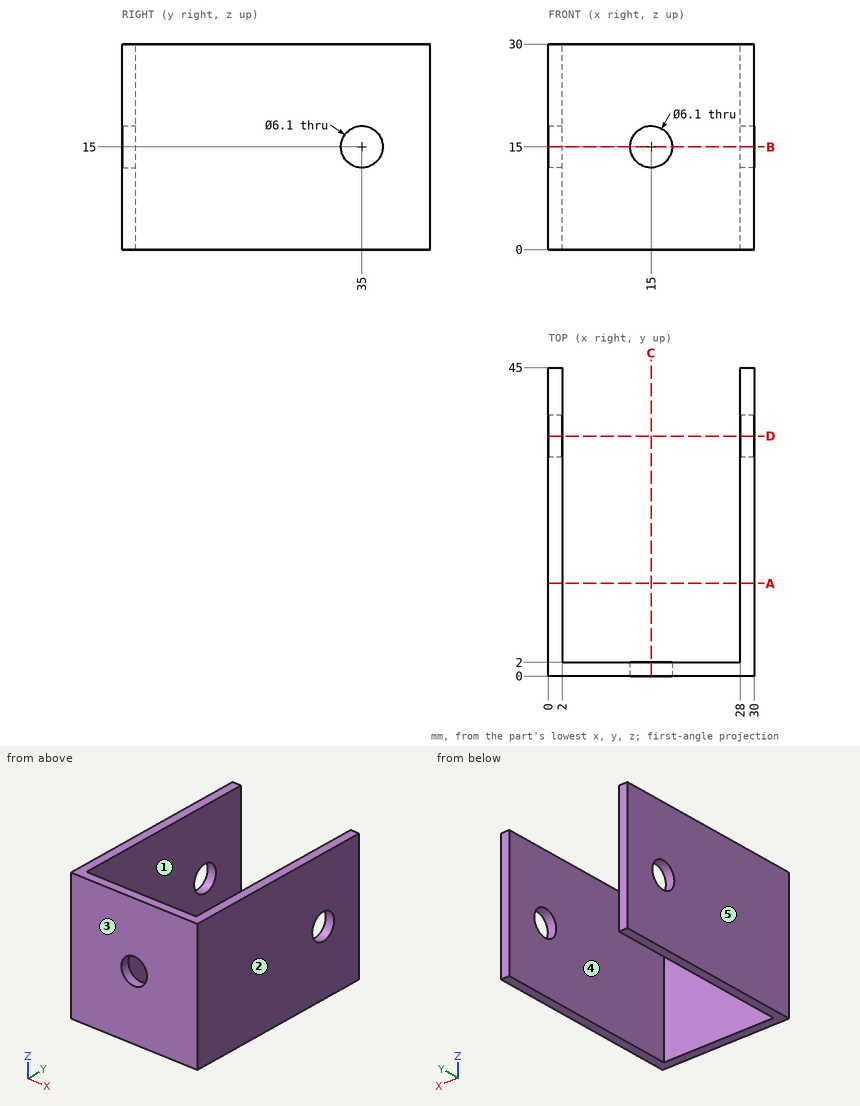
Source: three-view drawing plus pictorial views. Frame: mm from the lowest corner of the part. A direction names the side the tool comes from. Coordinates: 2 decimals unless noted, no trailing zeros. Loops run counter-clockwise (first coordinate to the right, second up) from the corner with the lowest first, then second, coordinate; pieces in that order, holes last. Notation, with made-up numbers: (25.5, 13.25) - (60.5, 13.25) arc R15 cw to (60.5, 29.25) - close; hole circle Ø11 at (78.25, 82.5). An arc over 180 degrees is marked (long way). One line per item, written item: value. Start each with the question number.
1. Section D-D (y = 35). Return the cut outline in (x, z), and give its area (3 significant figures).
2. Section C-C (x = 15). Return the cut outline in (y, z).
3. Mould query, pull axis X, two halves, no side actions, for the marked faces 1, 2 and 3. Classes: pulls with the +X half, pulls with the -X half, needs draft (parallel to the pull), parting line crosses it, or undercut.
4. Section A-A (y = 13.5). Return the cut outline in (x, z).
5. Ray query, L1, parallel to X at y = 43, z = 5.75; L2, parallel to Z at x = 15, y = 0.4. Return the intervals inside material, ascending.
6. Contact query for flat-ended pins moving along their axis: P1, Ø13, axis at x = 19.5, z = 13.5, coming from the +Y side; P2, Ø5, axis at x = 15, z = 15, coming from the +Y side. Output: stop coordinate, or through.
7. Set-up query: the marked faces 4 and 5. Return all of +Z, -Z, +X, -X, +Y, -Y with unobstructed straight access to the full face (end or side cutting, diameter ignored); none if empty.
8. Section B-B (z = 15). Return the cut outline in (x, y).
Verdict:
1. outline: (0, 0) - (2, 0) - (2, 11.95) - (0, 11.95) - close; (0, 18.05) - (2, 18.05) - (2, 30) - (0, 30) - close; (28, 0) - (30, 0) - (30, 11.95) - (28, 11.95) - close; (28, 18.05) - (30, 18.05) - (30, 30) - (28, 30) - close
1. area: 95.6 mm2
2. outline: (0, 0) - (2, 0) - (2, 11.95) - (0, 11.95) - close; (0, 18.05) - (2, 18.05) - (2, 30) - (0, 30) - close
3. face 1: undercut
3. face 2: pulls with the +X half
3. face 3: needs draft
4. outline: (0, 0) - (2, 0) - (2, 30) - (0, 30) - close; (28, 0) - (30, 0) - (30, 30) - (28, 30) - close
5. L1: x = 0 to 2, 28 to 30
5. L2: z = 0 to 11.95, 18.05 to 30
6. P1: stops at y = 2
6. P2: passes through
7. face 4: +Z, -Z, +Y
7. face 5: +Z, -Z, -X, +Y, -Y
8. outline: (0, 0) - (11.95, 0) - (11.95, 2) - (2, 2) - (2, 31.95) - (0, 31.95) - close; (0, 38.05) - (2, 38.05) - (2, 45) - (0, 45) - close; (18.05, 0) - (30, 0) - (30, 31.95) - (28, 31.95) - (28, 2) - (18.05, 2) - close; (28, 38.05) - (30, 38.05) - (30, 45) - (28, 45) - close
